For this review, take the finished solid that the model builds, in its own axes (mm). A direction names the side the tool comes from. Round coordinates to 2 decimals unless told otherwise and drop trailing zeros. Order: outer loops, then holes, each group sorted by start corner. A loop starts at its lowest first (then second) coordinate and runs counter-clockwise, first axis right, second up. Notation, with made-up numbers: (49.5, 22.25) - (62.5, 22.25) arc R17 cw to (62.5, 51.25) - close; hole circle Ø4 at (89.25, 74). An arc over 180 degrees is marked (long way). Write each question's results on one line, items separated by ' | '. Start each with the question number.
(1) Draft analysis for pull direction Y (two halves, no side actions). For faces 1 (the cylindrical face through (158.336, 152.925, 86.275)), 2 (the flat face through (114, 8, 86)), 3 (the flat face through (79.105, 4, 86)), 4 (the cylindrical face through (-9.4, 3.85, 86.28)), state which applies: pulls with the +Y half, pulls with the -Y half, needs draft (parallel to the pull), parting line crosses it, or undercut.
(2) For L1, parallel to X at y = 143, z = 107; L2, parallel to X at y = 18, z = 159.5; L3, parallel to X at y = 140, z = 115, list the stretches that pass through material, from the lowest coordinate up. Write a range as from..to.
(3) Take a section at B-B, the plane z = 102.5. Give the boundary of the cut face in (x, y), plus the area to 3 significant figures.
(4) Take a section at A-A, the plane y = 39.5. Give the boundary of the cut face in (x, z), plus the area to 3 significant figures.
(5) Take a section at C-C, the plane x = 153. Give the boundary of the cut face in (y, z).
(6) Insertion check: pin 1 Ø3 at (x, z) = (86.5, 68) entering from +Y; pin 2 Ø2.5 at (y, z) = (4.5, 93) entering from -X (3 decimals); pin 3 Ø10 at (x, z) = (115, 84.5) entering from +Y. Each pin has a flat end and moves straight along its axis. Give the tip position at first contact, or say it passes through.
(7) Take a section at D-D, the plane x = 43. Give the boundary of the cut face in (y, z), plus the area to 3 significant figures.
(8) For faces 5 (the flat face through (-2.806, 22.001, 86.275)), 6 (the flat face through (77.89, 73.08, 86.28)), 7 (the flat face through (76, 72, 175)), list the 3-axis set-ups (+Z, -Z, +X, -X, +Y, -Y) from which the entire face can be reached by the end or side of a thin tool; tool diameter is ignored.
```python
from build123d import *

# Parameters (mm, degrees)
PAD002_DEPTH = 175


with BuildPart() as part:
    # Sketch → Pad002 (new body)
    with BuildSketch(Plane.XY):
        with BuildLine():
            Line((8.468198, 3.655669), (149.280288, 144.467759))
            ThreePointArc((158.352585, 140.709891), (155.0719, 145.619782), (149.280288, 144.467759))
            Line((158.352585, 140.709891), (158.352585, 18.903732))
            ThreePointArc((147.448852, 8), (155.158955, 11.193629), (158.352585, 18.903732))
            Line((147.448852, 8), (79.105045, 8))
            Line((79.105045, 8), (79.105045, 0))
            Line((79.105045, 0), (147.448852, 0))
            ThreePointArc((147.448852, 0), (160.81581, 5.536775), (166.352585, 18.903732))
            Line((166.352585, 18.903732), (166.352585, 140.709891))
            ThreePointArc((166.352585, 140.709891), (158.133368, 153.010819), (143.623434, 150.124613))
            Line((143.623434, 150.124613), (2.202078, 8.703257))
            Line((-4.161883, 15.067218), (2.202078, 8.703257))
            Line((-4.161883, 15.067218), (-0.017083, 19.212018))
            Line((-0.017083, 19.212018), (-5.673937, 24.868873))
            Line((-5.673937, 24.868873), (-9.209471, 21.333339))
            ThreePointArc((-9.209471, 21.333339), (-9.209471, 3.655669), (8.468198, 3.655669))
        make_face()
    extrude(amount=PAD002_DEPTH)


solid = part.part
```
Results below:
1) face 1: pulls with the +Y half | face 2: undercut | face 3: needs draft | face 4: parting line crosses it
2) L1: x = 136.5..147.81, 157.83..166.15 | L2: x = -11.59..-1.23, 11.5..22.81, 158.32..166.33 | L3: x = 133.5..144.81, 158.35..166.35
3) outline: (-9.21, 21.33) arc R12.5 ccw to (8.47, 3.66) - (149.28, 144.47) arc R5.31 cw to (158.35, 140.71) - (158.35, 18.9) arc R10.9 cw to (147.45, 8) - (79.11, 8) - (79.11, 0) - (147.45, 0) arc R18.9 ccw to (166.35, 18.9) - (166.35, 140.71) arc R13.31 ccw to (143.62, 150.12) - (2.2, 8.7) - (-4.16, 15.07) - (-0.02, 19.21) - (-5.67, 24.87) - close | area: 3,750 mm^2
4) outline: (33, 0) - (44.31, 0) - (44.31, 175) - (33, 175) - close; (158.35, 0) - (166.35, 0) - (166.35, 175) - (158.35, 175) - close | area: 3,380 mm^2
5) outline: (0.83, 0) - (9.52, 0) - (9.52, 175) - (0.83, 175) - close; (146.02, 0) - (154.02, 0) - (154.02, 175) - (146.02, 175) - close
6) pin 1: stops at y = 94.5 | pin 2: stops at x = -10.895 | pin 3: stops at y = 126.5
7) outline: (38.19, 0) - (49.5, 0) - (49.5, 175) - (38.19, 175) - close | area: 1,980 mm^2
8) face 5: +Z, -Z, +Y | face 6: +Z, -Z | face 7: +Z, +X, -X, +Y, -Y
